Check sheet for the drawn part. Datum: minimum x, y, z corner. Units: mm. A direction names the side the tool comes from. Round coordinates to 2 decimals unless told otherwise and drop trailing zeros. Write each loop counter-clockwise with the first axis right and the second up, starting at its lowest first coordinate (ties: lowest second). Pieces come first, ordered by that corner, then holes. Notation, with made-up numbers: (55.5, 24) -> (94.5, 24) arc R6 ccw to (94.5, 31) -> close; hole circle Ø9 at (70.25, -7). An arc over 180 degrees is marked (long way). One line per item, written item: value.
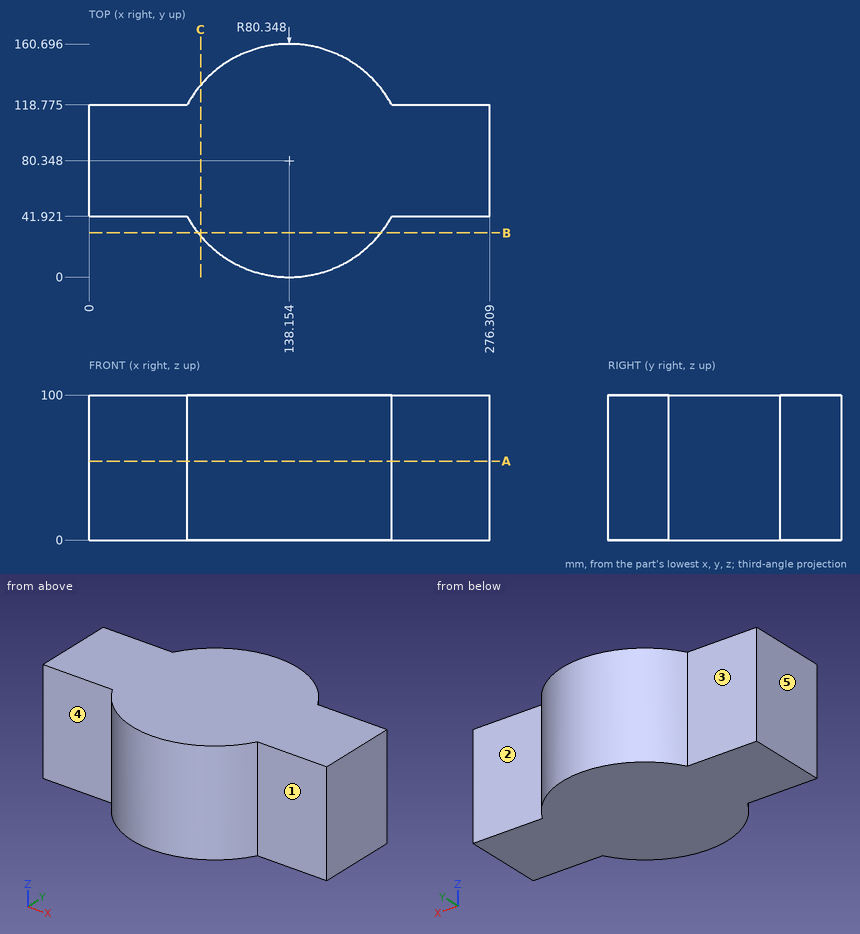
Item 1: Thickness scan on line 1 (Y direction, x = 25.5, z = 67.5) (1 decimal); line 2 (Y direction, x = 129, z = 76); line 3 (X direction, y = 141.5, z = 86.5) (1 decimal). Record the ranges inside material, lowest first.
Answer:
line 1: y = 41.9 to 118.8
line 2: y = 0.52 to 160.17
line 3: x = 86 to 190.3
Item 2: Sectioned sample at A-A on z = 54.5. Enter the section's corners in (x, y) (1 decimal).
Answer:
outline: (0, 41.9) -> (67.6, 41.9) arc R80.3 ccw to (208.7, 41.9) -> (276.3, 41.9) -> (276.3, 118.8) -> (208.7, 118.8) arc R80.3 ccw to (67.6, 118.8) -> (0, 118.8) -> close
Item 3: Depth check by flat-ended pin: P1, Ø1, axis at x = 186.5, z = 22.5, coming from the -Y side; P2, Ø1, axis at y = 40.5, z = 30.5, coming from the -X side; P3, Ø1.5, axis at y = 119, z = 42.5, coming from the -X side; P4, Ø5, axis at y = 30.5, z = 27, coming from the +X side. Enter the tip coordinate at first touch or a pass-through.
Answer:
P1: stops at y = 15.8
P2: stops at x = 68.1
P3: stops at x = 0
P4: stops at x = 203.07
Item 4: Sectioned sample at C-C on x = 77. Enter the section's corners in (y, z), and give its area (3 significant figures).
Answer:
outline: (28.23, 0) -> (132.46, 0) -> (132.46, 100) -> (28.23, 100) -> close
area: 10,400 mm^2
Item 5: Sectioned sample at B-B on y = 30.5. Enter the section's corners in (x, z), and give its area (3 significant figures).
Answer:
outline: (75.14, 0) -> (201.17, 0) -> (201.17, 100) -> (75.14, 100) -> close
area: 12,600 mm^2
Item 6: Tool access check on the marked faces 1, 2, 3, 4 and 5. Record the directions out of +Z, -Z, +X, -X, +Y, -Y that give a thin tool (end or side, any length) a straight path to the whole face; none if there is none.
Answer:
face 1: +Z, -Z, +X, -Y
face 2: +Z, -Z, +X, +Y
face 3: +Z, -Z, -X, +Y
face 4: +Z, -Z, -X, -Y
face 5: +Z, -Z, -X, +Y, -Y
